The listing builds one solid part. Answer for the finished solid, in the listing's coordinates (mm). A direction names the side the tool comes from. Round coordinates to 2 decimals unless told otherwise and drop trailing zeros. Write each loop counter-clockwise with the first axis right and the second up, starting at its lowest first coordinate (ties: lowest second). Pieces come first, ordered by that corner, then holes. Notation, with made-up numbers: (60.25, 8) - (109.25, 8) arc R7 ccw to (109.25, 17) - close; hole circle Ø4 at (-3.5, -4.5). An arc over 180 degrees is marked (long way). Answer in a Markdown table with one row per item.
from build123d import *

# Parameters (mm, degrees)
F1_DEPTH = 20


# Not quite as in the source:
# - ends of sketch curves that miss each other by under 0.0002 mm in the source are joined


with BuildPart() as f1:
    # F0 (on Front) → F1 (new body)
    with BuildSketch(Plane.XZ):
        with BuildLine():
            Line((97.2907843779, 1.1145511836), (34.0001858397, 10.009464731))
            Line((34.0001858397, 10.009464731), (33.8270701172, 10.0337945591))
            Line((33.8270701172, 10.0337945591), (33.7396616023, 10.0337945591))
            Line((33.7396616023, 10.0337945591), (-46.2468009406, 10.0337945591))
            ThreePointArc((-46.2468009406, 10.0337945591), (-57.7296417452, -0.9784425912), (-46.7174045949, -12.4612833958))
            Line((-46.7174045949, -12.4612833958), (33.1437814598, -12.4612833958))
            Line((33.1437814598, -12.4612833958), (87.1445596341, -25.8231245195))
            ThreePointArc((87.1445596341, -25.8231245195), (109.0413090103, -18.6910027208), (97.2907843779, 1.1145511836))
        make_face()
        with BuildLine():
            ThreePointArc((-46.7038671765, -11.2112851433), (-56.4796434927, -0.9919800096), (-46.260338359, 8.7837963066))
            Line((-46.260338359, 8.7837963066), (33.7396616023, 8.7837945591))
            Line((33.7396616023, 8.7837945591), (97.1168180017, -0.1232839023))
            ThreePointArc((97.1168180017, -0.1232839023), (107.8343480434, -18.3479856965), (87.6567253878, -24.6621562401))
            Line((87.6567253878, -24.6621562401), (33.2961328623, -11.2112833958))
            Line((33.2961328623, -11.2112833958), (-46.7038671765, -11.2112851433))
        make_face(mode=Mode.SUBTRACT)
    extrude(amount=F1_DEPTH)


solid = f1.part
(1) Flat-ended cylindrical pins translate along their axes: pin 1 (12 mm diameter, centred on x = 53, z = -17.5, fed in from -Y); pin 2 (12 mm diameter, centred on x = -16.5, y = -7.5, fed in from +Z); pin 3 (3 mm diameter, centred on x = -27.5, y = -2, fed in from -Z); pin 4 (6 mm diameter, centred on y = -11, z = 1.5, fed in from +X). Find the tip coordinate at first contact, or state that the pin passes through.
Checked values:
| item | result |
|---|---|
| pin 1 | stops at y = -20 |
| pin 2 | stops at z = 10.03 |
| pin 3 | stops at z = -12.46 |
| pin 4 | stops at x = 103.83 |
(2) Find the intervals of material crossed by line 1 (Z direction, x = 9.5, y = -11); line 2 (Z direction, x = 65, y = -14.25); line 3 (X direction, y = -9.75, z = -8), in increasing order.
Checked values:
| item | result |
|---|---|
| line 1 | z = -12.46 to -11.21, 8.78 to 10.03 |
| line 2 | z = -20.34 to -19.06, 4.39 to 5.65 |
| line 3 | x = -55.45 to -53.83, 107.57 to 108.93 |
(3) Section A-A (x = 0) is taken. Give the vertices of the cut face in (y, z), and give its area (3 significant figures).
Checked values:
| item | result |
|---|---|
| outline | (-20, -12.46) - (0, -12.46) - (0, -11.21) - (-20, -11.21) - close; (-20, 8.78) - (0, 8.78) - (0, 10.03) - (-20, 10.03) - close |
| area | 50.0 mm2 |
(4) For faces 4 (the flat face through (26, -20, -12)), 5 (the flat face through (-6, -10, -11.211)), 6 (the flat face through (-7, -10, -12.461)), determine the directions among +Z, -Z, +X, -X, +Y, -Y from which every point of the face is accessible in a straight line to the end or side of a thin tool.
Checked values:
| item | result |
|---|---|
| face 4 | +Z, -Z, +X, -X, -Y |
| face 5 | +Y, -Y |
| face 6 | -Z, -X, +Y, -Y |
(5) Section C-C (z = -23) is taken. Give the vertices of the cut face in (x, y), and give its area (3 significant figures).
Checked values:
| item | result |
|---|---|
| outline | (75.74, -20) - (80.94, -20) - (80.94, 0) - (75.74, 0) - close; (104.82, -20) - (106.51, -20) - (106.51, 0) - (104.82, 0) - close |
| area | 138 mm2 |
(6) For a pull along X with two mould halves and no side action, classify faces 1 (the cylindrical face through (-56.482, -9.86, -1.212)), 2 (the flat face through (26, 0, -12)), 3 (the flat face through (59.77, -9.86, -19.05)) as pulls with the +X half, pulls with the -X half, needs draft (parallel to the pull), parting line crosses it, or undercut.
Checked values:
| item | result |
|---|---|
| face 1 | undercut |
| face 2 | needs draft |
| face 3 | pulls with the -X half |
(7) Section B-B (y = -13) is taken. Give the vertices of the cut face in (x, z), and give its area (3 significant figures).
Checked values:
| item | result |
|---|---|
| outline | (-46.72, -12.46) - (33.14, -12.46) - (87.14, -25.82) arc R14.75 ccw (long way) to (97.29, 1.11) - (33.83, 10.03) - (-46.25, 10.03) arc R11.25 ccw to start; hole (-46.7, -11.21) - (33.3, -11.21) - (87.66, -24.66) arc R13.5 ccw (long way) to (97.12, -0.12) - (33.74, 8.78) - (-46.26, 8.78) arc R10 ccw to start |
| area | 455 mm2 |
